The model under review builds one solid part; all positions refer to its coordinate system, in mm. Face numbers are marked on the shaded views. Coordinates: 2 decimals unless noted, no trailing zeros. Order: outer loops, then holes, each group sorted by start corner. A loop starts at its lowest first (then second) coordinate and runs counter-clockwise, first axis right, second up. Notation, with made-up numbers: M 25,81 L 54,81 A27 cw 54,103 Z; hole C -18.75,-28.5 d2. An arc over 180 degrees is marked long. One line per item, written item: value.
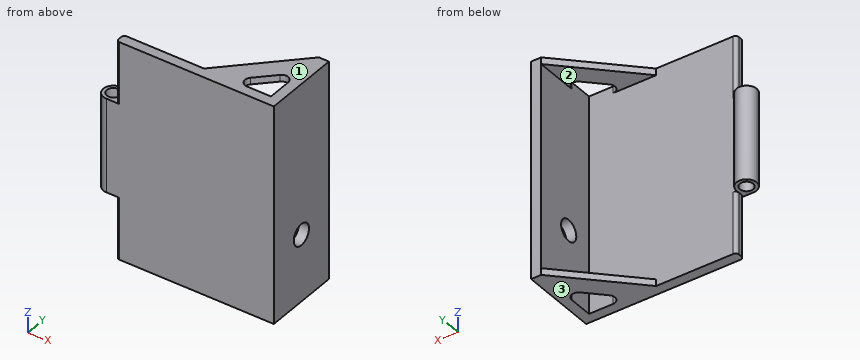
```python
from build123d import *

# Parameters (mm, degrees)
SKETCH1_W           = 50
SKETCH1_H           = 65
BOSS_EXTRUDE1_DEPTH = 3
SKETCH2_W           = 3
SKETCH2_H           = 3
CUT_EXTRUDE1_DEPTH  = 18.5
SKETCH3_W           = 3
SKETCH3_H           = 3
CUT_EXTRUDE2_DEPTH  = 18.5
SKETCH4_R           = 3
BOSS_EXTRUDE2_DEPTH = 28
SKETCH5_R           = 2
CUT_EXTRUDE3_DEPTH  = 28
FILLET1_R           = 1
SKETCH6_W           = 3
SKETCH6_H           = 65
BOSS_EXTRUDE3_DEPTH = 20
BOSS_EXTRUDE4_DEPTH = 2
BOSS_EXTRUDE5_DEPTH = 2
CUT_EXTRUDE4_DEPTH  = 82
FILLET2_R           = 2
SKETCH10_R          = 3.175
CUT_EXTRUDE5_DEPTH  = 82


with BuildPart() as part:
    # Sketch1 → Boss-Extrude1 (new body)
    with BuildSketch(Plane(origin=(0, 0, 0), x_dir=(1, 0, 0), z_dir=(0, 1, 0))):
        Rectangle(SKETCH1_W, SKETCH1_H)
    extrude(amount=BOSS_EXTRUDE1_DEPTH)

    # Sketch2 → Cut-Extrude1 (cut)
    with BuildSketch(Plane.XY.offset(32.5)):
        with Locations((-23.5, 1.5)):
            Rectangle(SKETCH2_W, SKETCH2_H)
    extrude(amount=-CUT_EXTRUDE1_DEPTH, mode=Mode.SUBTRACT)

    # Sketch3 → Cut-Extrude2 (cut)
    with BuildSketch(Plane(origin=(0, 0, -32.5), x_dir=(-1, 0, 0), z_dir=(0, 0, -1))):
        with Locations((23.5, 1.5)):
            Rectangle(SKETCH3_W, SKETCH3_H)
    extrude(amount=-CUT_EXTRUDE2_DEPTH, mode=Mode.SUBTRACT)

    # Sketch4 → Boss-Extrude2 (add)
    with BuildSketch(Plane.XY.offset(14)):
        with Locations((-25, 3)):
            Circle(SKETCH4_R)
    extrude(amount=-BOSS_EXTRUDE2_DEPTH)

    # Sketch5 → Cut-Extrude3 (cut)
    with BuildSketch(Plane.XY.offset(14)):
        with Locations((-25, 3)):
            Circle(SKETCH5_R)
    extrude(amount=-CUT_EXTRUDE3_DEPTH, mode=Mode.SUBTRACT)

    # Fillet1
    fillet1_edges = [part.edges().sort_by_distance(p)[0] for p in [
        (-22, 3, 23.25),
        (-22, 0, 23.25),
        (-22, 0, -23.25),
        (-22, 3, -23.25),
    ]]
    fillet(fillet1_edges, radius=FILLET1_R)

    # Sketch6 → Boss-Extrude3 (add)
    with BuildSketch(Plane(origin=(0, 3, 0), x_dir=(1, 0, 0), z_dir=(0, 1, 0))):
        with Locations((23.5, 0)):
            Rectangle(SKETCH6_W, SKETCH6_H)
    extrude(amount=BOSS_EXTRUDE3_DEPTH)

    # Sketch7 → Boss-Extrude4 (add)
    with BuildSketch(Plane.XY.offset(32.5)):
        Polygon((22, 23), (22, 3), (2, 3), align=None)
    extrude(amount=-BOSS_EXTRUDE4_DEPTH)

    # Sketch8 → Boss-Extrude5 (add)
    with BuildSketch(Plane(origin=(0, 0, -32.5), x_dir=(-1, 0, 0), z_dir=(0, 0, -1))):
        Polygon((-22, 23), (-2, 3), (-22, 3), align=None)
    extrude(amount=-BOSS_EXTRUDE5_DEPTH)

    # Sketch9 → Cut-Extrude4 (cut)
    with BuildSketch(Plane.XY.offset(32.5)):
        Polygon((22, 15), (22, 3), (10, 3), align=None)
    extrude(amount=-CUT_EXTRUDE4_DEPTH, mode=Mode.SUBTRACT)

    # Fillet2
    fillet2_edges = [part.edges().sort_by_distance(p)[0] for p in [
        (10, 3, -31.5),
        (22, 15, -31.5),
        (10, 3, 31.5),
        (22, 15, 31.5),
    ]]
    fillet(fillet2_edges, radius=FILLET2_R)

    # Sketch10 → Cut-Extrude5 (cut)
    with BuildSketch(Plane(origin=(25, 0, 0), x_dir=(0, 0, -1), z_dir=(1, 0, 0))):
        with Locations((12.5, 11.5)):
            Circle(SKETCH10_R)
    extrude(amount=-CUT_EXTRUDE5_DEPTH, mode=Mode.SUBTRACT)


solid = part.part
```
(1) We need section D-D, the plane z = -21. State the section outline as (x, y) points, plus the area to 3 significant figures.
Geometry results:
outline: M -22,1 A1 ccw -21,0 L 25,0 L 25,23 L 22,23 L 22,3 L -21,3 A1 ccw -22,2 Z
area: 201 mm2
(2) Insertion check: pin 1 Ø3 at (y, z) = (16.5, 17) entering from -X; pin 2 Ø6 at (x, y) = (8.5, 14) entering from -Z; pin 3 Ø5 at (x, y) = (-25, 3) entering from +Z; pin 4 Ø1.1 at (y, z) = (1.5, 27) entering from -X. Each pin has a flat end and moves straight along its axis. Give the tip position at first contact, or say it passes through.
Geometry results:
pin 1: stops at x = 22
pin 2: passes through
pin 3: stops at z = 14
pin 4: stops at x = -22
(3) For L1, parallel to Y at x = -25, z = 7; L2, parallel to Z at x = 9, y = 6.75; L3, parallel to Y at x = -15.5, z = 9.5, list the stretches that pass through material, from the lowest coordinate up.
Geometry results:
L1: y = 0 to 1, 5 to 6
L2: z = -32.5 to -30.5, 30.5 to 32.5
L3: y = 0 to 3
(4) We need section A-A, the plane z = -12.5. State the section outline as (x, y) points (3 decimals).
Geometry results:
outline: M -25,0 L 25,0 L 25,8.325 L 22,8.325 L 22,3 L -22,3 A3 ccw long Z; M 22,14.675 L 25,14.675 L 25,23 L 22,23 Z; hole C -25,3 d4
(5) Mouldability with a two-part tool opening along Z and no side actions: class the marked faces 1, 2 and 3 as +Z half, -Z half, draft (parallel to the pull), parting line (faces both ways), or undercut.
Geometry results:
face 1: +Z half
face 2: undercut
face 3: -Z half
(6) We need section C-C, the plane x = 11.5. State the section outline as (y, z) points.
Geometry results:
outline: M 0,-32.5 L 12.5,-32.5 L 12.5,-30.5 L 3,-30.5 L 3,30.5 L 12.5,30.5 L 12.5,32.5 L 0,32.5 Z
(7) We need section B-B, the plane y = 13. State the section outline as (x, z) points, plus the area to 3 significant figures.
Geometry results:
outline: M 12,-32.5 L 25,-32.5 L 25,-15.3 L 22,-15.3 L 22,-30.5 L 12,-30.5 Z; M 12,30.5 L 22,30.5 L 22,-9.7 L 25,-9.7 L 25,32.5 L 12,32.5 Z
area: 218 mm2
